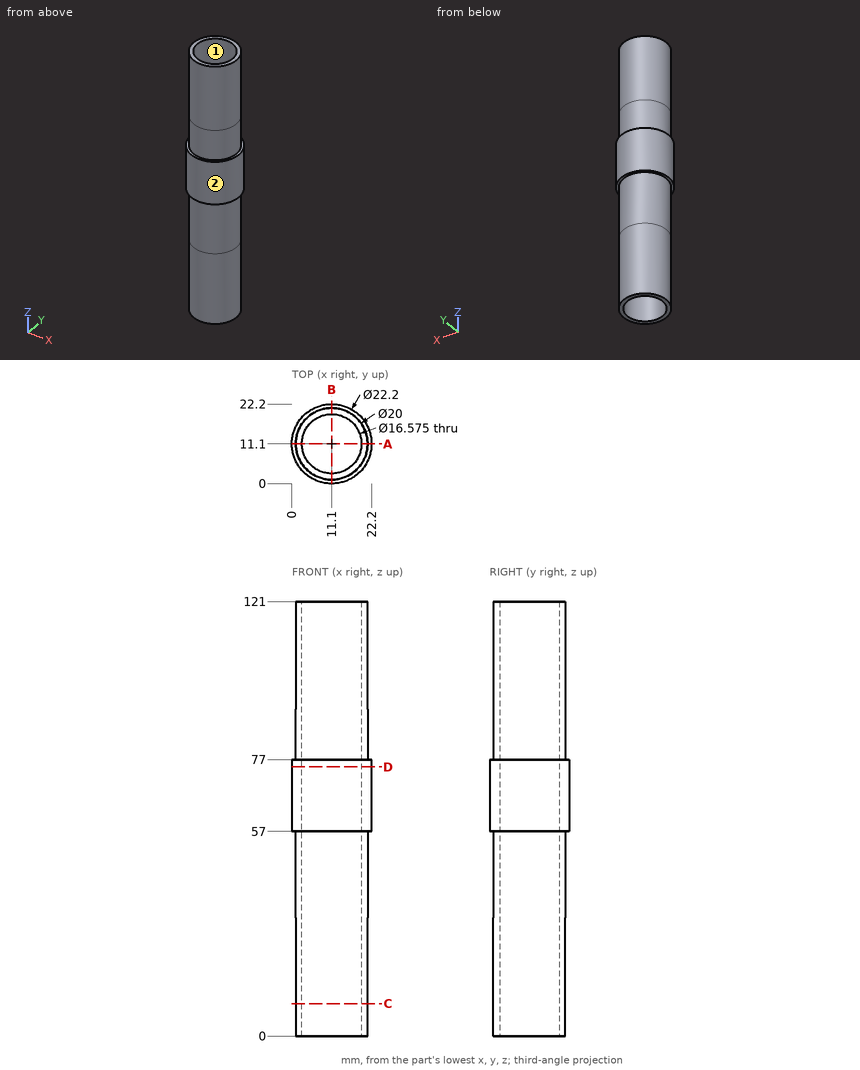
Check sheet for the drawn part. Datum: minimum x, y, z corner. Units: mm. Coordinates: 2 decimals unless noted, no trailing zeros. Order: outer loops, then holes, each group sorted by start corner. A loop starts at its lowest first (then second) coordinate and runs counter-clockwise, first axis right, second up. Notation, with made-up numbers: (2.5, -5) -> (24.5, -5) arc R23 ccw to (24.5, 16) -> close; hole circle Ø6 at (32, -10). An arc over 180 degrees is marked (long way). Write each question's results on one line, items separated by ' | '. Start each with the question number.
1) Section check A-A (y = 11.1). Enter the section's corners in (x, z).
2) Section check D-D (z = 75). Enter the section's corners in (x, y) (1 decimal), and give its area (3 significant figures).
3) Material ranges on line 1 along Y through (x, z) = (11.1, 95.5); line 2 along X through (y, z) = (10.75, 62.5); line 3 along X through (y, z) = (16, 13), recorded low to high.
4) Depth check by flat-ended pin: pin 1 (11 mm diameter, centred on x = 11.5, y = 11, fed in from -Z); pin 2 (8 mm diameter, centred on y = 10, z = 62.5, fed in from -X); pin 3 (1.5 mm diameter, centred on y = 14.5, z = 83.5, fed in from +X); pin 4 (8 mm diameter, centred on x = 17.5, z = 43, fed in from +Y). Enter the tip coordinate at first touch or a pass-through.
5) Section check C-C (z = 9). Enter the section's corners in (x, y) (1 decimal).
6) Draft check along Y on the marked faces 1 and 2. Enter one of: pulls with the +Y half, pulls with the -Y half, needs draft (parallel to the pull), parting line crosses it, or undercut.
Checked values:
1) outline: (0, 57) -> (1.1, 57) -> (1.1, 0) -> (2.81, 0) -> (2.81, 121) -> (1.1, 121) -> (1.1, 77) -> (0, 77) -> close; (19.39, 0) -> (21.1, 0) -> (21.1, 57) -> (22.2, 57) -> (22.2, 77) -> (21.1, 77) -> (21.1, 121) -> (19.39, 121) -> close
2) outline: circle Ø22.2 at (11.1, 11.1); hole circle Ø16.6 at (11.1, 11.1) | area: 171 mm²
3) line 1: 1.1 to 2.81, 19.39 to 21.1 | line 2: 0.01 to 2.82, 19.38 to 22.19 | line 3: 2.38 to 4.42, 17.78 to 19.82
4) pin 1: through | pin 2: x = 0 | pin 3: x = 20.74 | pin 4: y = 20.81
5) outline: circle Ø20 at (11.1, 11.1); hole circle Ø16.6 at (11.1, 11.1)
6) face 1: undercut | face 2: parting line crosses it
